Verification items for the finished model (mm, model axes). Face numbers are marked on the shaded views. A direction names the side the tool comes from. Coordinates: 2 decimals unless noted, no trailing zeros. Write each loop counter-clockwise with the first axis right and the second up, starting at its lowest first coordinate (ties: lowest second). Pieces come first, ordered by that corner, then holes.
```python
from build123d import *

# Parameters (mm, degrees)
SKETCH1_W            = 60
SKETCH1_H            = 68
BOSS_EXTRUDE1_DEPTH  = 7
M4_CLEARANCE_HOLE4_D = 4.5
CUT_EXTRUDE5_DEPTH   = 91.956033335
FILLET3_R            = 10
SKETCH30_W           = 68
SKETCH30_H           = 7
BOSS_EXTRUDE8_DEPTH  = 5
SKETCH31_W           = 7
SKETCH31_H           = 68
BOSS_EXTRUDE9_DEPTH  = 25
M4_CLEARANCE_HOLE5_D = 4.5
BOSS_EXTRUDE12_DEPTH = 3
BOSS_EXTRUDE13_DEPTH = 3


with BuildPart() as part:
    # Sketch1 → Boss-Extrude1 (new body)
    with BuildSketch(Plane(origin=(0, 0, 0), x_dir=(1, 0, 0), z_dir=(0, 1, 0))):
        with Locations((30, 34)):
            Rectangle(SKETCH1_W, SKETCH1_H)
    extrude(amount=BOSS_EXTRUDE1_DEPTH)

    # M4 Clearance Hole4 (through all)
    with Locations(Plane(origin=(0, 0, 0), x_dir=(-1, 0, 0), z_dir=(0, -1, 0))):
        with Locations((-50, 54), (-50, 14), (-10, 34)):
            Hole(M4_CLEARANCE_HOLE4_D / 2)

    # Sketch29 → Cut-Extrude5 (cut, through all)
    with BuildSketch(Plane.XZ):
        Polygon((39, 0), (27, -12), (17, -12), (0, -29), (0, 0), align=None)
        Polygon((0, -39), (0, -68), (39, -68), (27, -56), (17, -56), align=None)
    extrude(amount=-CUT_EXTRUDE5_DEPTH, mode=Mode.SUBTRACT)

    # Fillet3
    fillet3_edges = [part.edges().sort_by_distance(p)[0] for p in [
        (39, 3.5, 0),
        (27, 3.5, -12),
        (17, 3.5, -12),
        (0, 3.5, -29),
        (0, 3.5, -39),
        (17, 3.5, -56),
        (27, 3.5, -56),
        (39, 3.5, -68),
    ]]
    fillet(fillet3_edges, radius=FILLET3_R)

    # Sketch30 → Boss-Extrude8 (add)
    with BuildSketch(Plane(origin=(60, 0, 0), x_dir=(0, 0, -1), z_dir=(1, 0, 0))):
        with Locations((34, 3.5)):
            Rectangle(SKETCH30_W, SKETCH30_H)
    extrude(amount=BOSS_EXTRUDE8_DEPTH)

    # Sketch31 → Boss-Extrude9 (add)
    with BuildSketch(Plane.XZ):
        with Locations((61.5, -34)):
            Rectangle(SKETCH31_W, SKETCH31_H)
    extrude(amount=BOSS_EXTRUDE9_DEPTH)

    # M4 Clearance Hole5 (through all)
    with Locations(Plane(origin=(65, 0, 0), x_dir=(0, 0, -1), z_dir=(1, 0, 0))):
        with Locations((59, -6), (59, -18), (9, -6), (9, -18)):
            Hole(M4_CLEARANCE_HOLE5_D / 2)

    # Sketch36 → Boss-Extrude12 (add)
    with BuildSketch(Plane.XY):
        Polygon((58, -25), (43.142135624, 0), (58, 0), align=None)
    extrude(amount=-BOSS_EXTRUDE12_DEPTH)

    # Sketch37 → Boss-Extrude13 (add)
    with BuildSketch(Plane(origin=(0, 0, -68), x_dir=(-1, 0, 0), z_dir=(0, 0, -1))):
        Polygon((-43.142135624, 0), (-58, -25), (-58, 0), align=None)
    extrude(amount=-BOSS_EXTRUDE13_DEPTH)


solid = part.part
```
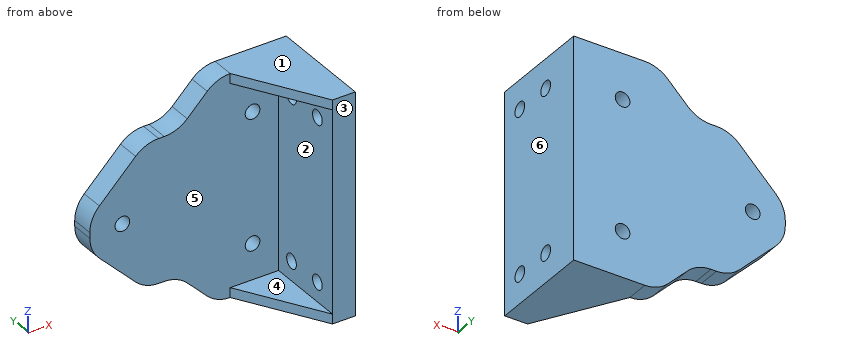
1. Sectioned sample at D-D, the plane y = -5. Record the boundary of the cut face in (x, z).
2. Gauge pin test, flat ends, axial feed: P1, Ø5, axis at x = 50, z = -54, coming from the +Y side; P2, Ø7, axis at y = -6, z = -9, coming from the -X side; P3, Ø3.5, axis at x = 50, z = -14, coming from the -Y side; P4, Ø1.9, axis at x = 21.5, y = 2.5, coming from the -Z side. Record the tip position at first contact, or that the pin passes through.
3. Sectioned sample at C-C, the plane x = 9. Record the boundary of the cut face in (y, z), and give its area (3 significant figures).
4. Tool access check on the marked faces 5 and 6. Record the directions out of +Z, -Z, +X, -X, +Y, -Y that give a thin tool (end or side, any length) a straight path to the whole face; none if there is none.
5. Sectioned sample at B-B, the plane y = 1. Record the boundary of the cut face in (x, z).
6. Material ranges on L1, parallel to Y at x = 60.25, z = -9; L2, parallel to Z at x = 50, y = 4.25; L3, parallel to X at y = 3.25, z = -34, recorded low to high.
7. Sectioned sample at A-A, the plane z = -34. Record the boundary of the cut face in (x, y), and give its area (4 significant figures).
8. Draft check along Z on the marked faces 1, 2, 3 and 4. Enter one of: pulls with the +Z half, pulls with the -Z half, needs draft (parallel to the pull), parting line crosses it, or undercut.
Outcome:
1. outline: (46.11, -68) - (65, -68) - (65, -61.02) - (58, -61.02) - (58, -65) - (46.11, -65) - close; (46.11, -3) - (58, -3) - (58, -6.98) - (65, -6.98) - (65, 0) - (46.11, 0) - close; (58, -56.98) - (65, -56.98) - (65, -11.02) - (58, -11.02) - close
2. P1: stops at y = 7
2. P2: stops at x = 58
2. P3: passes through
2. P4: stops at z = -56
3. outline: (0, -48) - (7, -48) - (7, -36.02) - (0, -36.02) - close; (0, -31.98) - (7, -31.98) - (7, -20) - (0, -20) - close
3. area: 168 mm2
4. face 5: -X, -Y
4. face 6: +Z, -Z, +X, +Y, -Y
5. outline: (0, -34.86) arc R10 ccw to (2.93, -41.93) - (14.07, -53.07) arc R10 ccw to (21.14, -56) - (22.86, -56) arc R10 cw to (29.93, -58.93) - (36.07, -65.07) arc R10 ccw to (43.14, -68) - (65, -68) - (65, 0) - (43.14, 0) arc R10 ccw to (36.07, -2.93) - (29.93, -9.07) arc R10 cw to (22.86, -12) - (21.14, -12) arc R10 ccw to (14.07, -14.93) - (2.93, -26.07) arc R10 ccw to (0, -33.14) - close; hole circle Ø4.5 at (10, -34); hole circle Ø4.5 at (50, -54); hole circle Ø4.5 at (50, -14)
6. L1: y = -25 to -20.25, -15.75 to -8.25, -3.75 to 7
6. L2: z = -68 to -56.25, -51.75 to -16.25, -11.75 to 0
6. L3: x = 0 to 7.75, 12.25 to 65
7. outline: (0, 0) - (7.75, 0) - (7.75, 7) - (0, 7) - close; (12.25, 0) - (58, 0) - (58, -25) - (65, -25) - (65, 7) - (12.25, 7) - close
7. area: 598.5 mm2
8. face 1: pulls with the +Z half
8. face 2: undercut
8. face 3: needs draft
8. face 4: undercut
